The figure shows three views and two pictorial views of one solid part (mm, origin at its lowest corner). Answer the questions. Round coordinates to 2 decimals unless told otherwise and drop trailing zeros. Order: outer loops, then holes, each group sorted by start corner. A loop starts at its lowest first (then second) coordinate and runs counter-clockwise, first axis right, second up.
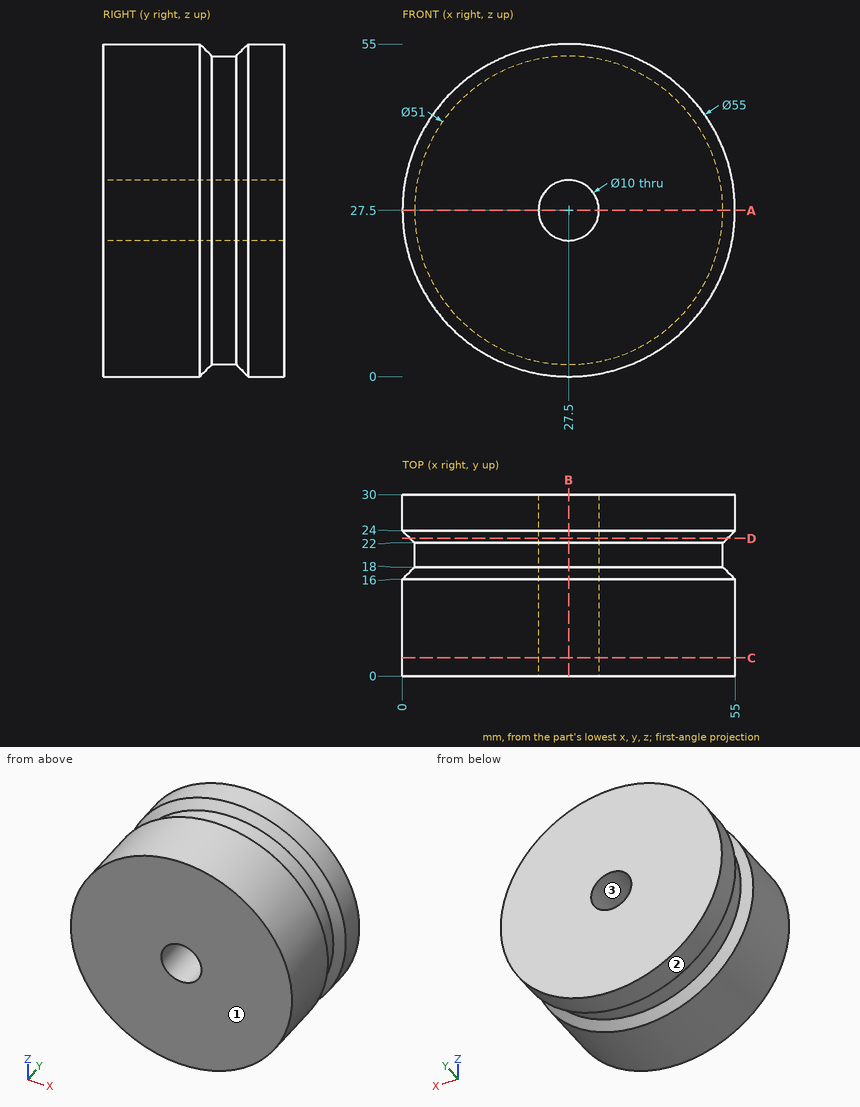
Item 1: Find the intervals of material crossed by line 1 along Z through (x, y) = (27.5, 7.5); line 2 along Z through (x, y) = (27.5, 21); line 3 along X through (y, z) = (13.5, 26), in increasing order.
Item 2: For a pull along X with two mould halves and no side action, classify the marked faces 1, 2 and 3 as released by +X, released by -X, zero draft, split by the parting line, or undercut.
Item 3: Find section B-B (x = 27.5). Write down the section's boundary in (y, z), plus the area to 3 significant figures.
Item 4: Given pin 1 (10 mm diameter, centred on y = 23.5, z = 16.5, fed in from -X); pin 2 (1.5 mm diameter, centred on y = 13, z = 25, fed in from +X); pin 3 (5 mm diameter, centred on y = 11, z = 9, fed in from -X); pin 4 (8 mm diameter, centred on x = 27.5, z = 27.5, fed in from +Y), each flat-ended and moving along its own axis, determine where each tip first touches the part or whether it passes through.
Item 5: Find section A-A (z = 27.5). Write down the section's boundary in (x, y), plus the area to 3 significant figures.
Item 6: Find section C-C (y = 3). Write down the section's boundary in (x, z), plus the area to 3 significant figures.
Item 7: Find section D-D (y = 22.75). Write down the section's boundary in (x, z).
Model answer:
1. line 1: z = 0 to 22.5, 32.5 to 55
1. line 2: z = 2 to 22.5, 32.5 to 53
1. line 3: x = 0.04 to 22.73, 32.27 to 54.96
2. face 1: zero draft
2. face 2: split by the parting line
2. face 3: undercut
3. outline: (0, 0) - (16, 0) - (18, 2) - (22, 2) - (24, 0) - (30, 0) - (30, 22.5) - (0, 22.5) - close; (0, 32.5) - (30, 32.5) - (30, 55) - (24, 55) - (22, 53) - (18, 53) - (16, 55) - (0, 55) - close
3. area: 1,330 mm2
4. pin 1: stops at x = 0.67
4. pin 2: stops at x = 54.94
4. pin 3: stops at x = 5.13
4. pin 4: passes through
5. outline: (0, 0) - (22.5, 0) - (22.5, 30) - (0, 30) - (0, 24) - (2, 22) - (2, 18) - (0, 16) - close; (32.5, 0) - (55, 0) - (55, 16) - (53, 18) - (53, 22) - (55, 24) - (55, 30) - (32.5, 30) - close
5. area: 1,330 mm2
6. outline: circle Ø55 at (27.5, 27.5); hole circle Ø10 at (27.5, 27.5)
6. area: 2,300 mm2
7. outline: circle Ø52.5 at (27.5, 27.5); hole circle Ø10 at (27.5, 27.5)
